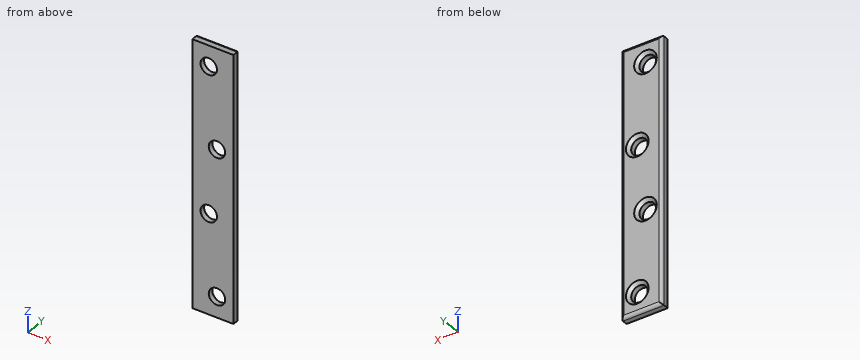
from build123d import *

# Parameters (mm, degrees)
SKETCH1_W           = 15.875
SKETCH1_H           = 101.6
BOSS_EXTRUDE1_DEPTH = 3.175
SKETCH2_R           = 3.175
CUT_EXTRUDE1_DEPTH  = 103.881758587
CHAMFER1_SIZE       = 1.190625
FILLET1_R           = 1.190625


with BuildPart() as part:
    # Sketch1 → Boss-Extrude1 (new body)
    with BuildSketch(Plane(origin=(0, 0, 0), x_dir=(1, 0, 0), z_dir=(0, 1, 0))):
        with Locations((7.9375, 50.8)):
            Rectangle(SKETCH1_W, SKETCH1_H)
    extrude(amount=BOSS_EXTRUDE1_DEPTH)

    # Sketch2 → Cut-Extrude1 (cut, through all)
    with BuildSketch(Plane(origin=(0, 3.175, 0), x_dir=(1, 0, 0), z_dir=(0, 1, 0))):
        with Locations(Location((6.35, 63.5, 0), (0, 0, 270))):
            Circle(SKETCH2_R)
        with Locations(Location((9.525, 93.6625, 0), (0, 0, 270))):
            Circle(SKETCH2_R)
        with Locations(Location((9.525, 38.1, 0), (0, 0, 270))):
            Circle(SKETCH2_R)
        with Locations(Location((6.35, 7.9375, 0), (0, 0, 270))):
            Circle(SKETCH2_R)
    extrude(amount=-CUT_EXTRUDE1_DEPTH, mode=Mode.SUBTRACT)

    # Chamfer1
    chamfer1_edges = [part.edges().sort_by_distance(p)[0] for p in [
        (6.35, 3.175, -66.675),
        (9.525, 3.175, -96.8375),
        (9.525, 3.175, -41.275),
        (6.35, 3.175, -11.1125),
    ]]
    chamfer(chamfer1_edges, length=CHAMFER1_SIZE)

    # Fillet1
    fillet1_edges = [part.edges().sort_by_distance(p)[0] for p in [
        (15.875, 3.175, -50.8),
        (7.9375, 3.175, -101.6),
        (0, 3.175, -50.8),
        (7.9375, 3.175, 0),
    ]]
    fillet(fillet1_edges, radius=FILLET1_R)


solid = part.part
Verification items for the finished model (mm, model axes). Coordinates: 2 decimals unless noted, no trailing zeros. Order: outer loops, then holes, each group sorted by start corner. A loop starts at its lowest first (then second) coordinate and runs counter-clockwise, first axis right, second up. Notation, with made-up numbers: M 75,-2.5 L 129,-2.5 A25 ccw 129,25.5 Z; hole C -13.5,-26 d6. An arc over 180 degrees is marked long. Return JSON: item names as keys, results as strings.
1) Cross-section at B-B, the plane y = 0.7. Count the separate pieces of the cut face and the enclosed holes in it, and give its area (3 significant figures).
Answer list:
{"separate pieces": "1", "enclosed holes": "4", "area": "1,490 mm2"}
2) Thickness scan on L1, parallel to X at y = 0.9, z = -63.5 (3 decimals); L2, parallel to X at y = 0.6, z = -38.1 (3 decimals); L3, parallel to Z at x = 3.75, y = 1.8. Record the ranges inside material, lowest first. Write a range as [from, to].
Answer list:
{"L1": "[0, 3.175], [9.525, 15.875]", "L2": "[0, 6.35], [12.7, 15.875]", "L3": "[-101.6, -65.32], [-61.68, -9.76], [-6.12, 0]"}
3) Cross-section at A-A, the plane z = -63.5. Record the boundary of the cut face in (x, y) (3 decimals).
Answer list:
{"outline": "M 0,0 L 3.175,0 L 3.175,1.984 L 1.984,3.175 L 1.191,3.175 A1.191 ccw 0,1.984 Z; M 9.525,0 L 15.875,0 L 15.875,1.984 A1.191 ccw 14.684,3.175 L 10.716,3.175 L 9.525,1.984 Z"}
4) Gauge pin test, flat end, axial feed: pin 1 (1 mm diameter, centred on x = 2.5, z = -19.5, fed in from -Y). Record the tip position at first contact, or that the pin passes through.
Answer list:
{"pin 1": "y = 0"}
